Work out the finished part from the listing and answer in its coordinate system (mm). Face numbers are marked on the shaded views. A direction names the side the tool comes from. Give positions to 0.01 mm unless a question says otherwise; leave off trailing zeros. Order: outer loops, then holes, each group sorted by start corner. A loop starts at its lowest first (then second) coordinate and runs counter-clockwise, first axis right, second up.
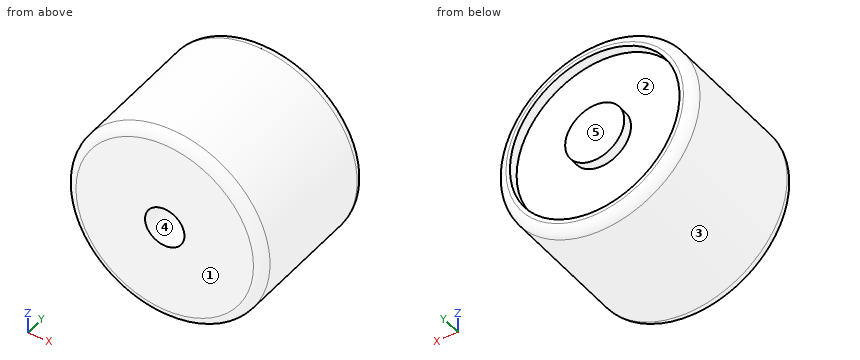
Autodesk Inventor part; units mm, degrees
ref_plane "YZ Plane" through (0, 0, 0) normal (1, 0, 0) x (0, 1, 0)
ref_plane "XZ Plane" through (0, 0, 0) normal (0, 1, 0) x (-1, 0, 0)
ref_plane "XY Plane" through (0, 0, 0) normal (0, 0, 1) x (1, 0, 0)
sketch "Boceto1" plane through (0, 0, 0) normal (0, 1, 0) x (-1, 0, 0)
  circle A0 centre (0, 0) radius 10
  dimension "d0" = 20
extrude "Extrusión1" add sketch "Boceto1" along normal blind 15
sketch "Boceto2" plane through (0, 15, 0) normal (0, 1, 0) x (1, 0, 0)
  circle A0 centre (0, 0) radius 3
  circle A1 centre (0, 0) radius 8.6
  circle A2 centre (0, 0) radius 10
  dimension "d3" = 1.4
  dimension "d4" = 6
extrude "Extrusión2" cut sketch "Boceto2" against normal blind 1 contours A1
sketch "Boceto3" plane through (0, 0, 0) normal (0, -1, 0) x (1, 0, 0)
  circle A0 centre (0, 0) radius 2
  dimension "d7" = 4
extrude "Extrusión3" cut sketch "Boceto3" against normal blind 7.5
fillet "Empalme1" radius 1 2 edges at (10, 0, 0) (10, 15, 0)
properties part number "electromagnet"
1. The part is cut by section D-D (y = 9). Write down the section's boundary in (x, z).
Findings below:
outline: circle Ø20 at (0, 0)
2. Straight lines are drawn through the part: probe 1 along Z at (x, y) = (0, 4.25); probe 2 along Z at (x, y) = (0, 14.7); probe 3 along X at (y, z) = (14.5, -6.25). For each, find the intervals that lie inside material, in ascending order.
Findings below:
probe 1: z = -10 to -2, 2 to 10
probe 2: z = -9.71 to -8.6, -3 to 3, 8.6 to 9.71
probe 3: x = -7.63 to -5.91, 5.91 to 7.63
3. The mould has two halves that part along X. Classify the marked faces 3, 4 and 5: pulls with the +X half, pulls with the -X half, needs draft (parallel to the pull), parting line crosses it, or undercut.
Findings below:
face 3: parting line crosses it
face 4: undercut
face 5: needs draft
4. Given P1, Ø1.5, axis at y = 11, z = 6, coming from the -X side; P2, Ø3, axis at y = 13.5, z = -7.5, coming from the -X side; P3, Ø1.5, axis at y = 11, z = -7, coming from the -X side; P4, Ø10, axis at x = -0.5, z = -6, coming from the +Y side, each flat-ended and moving along its own axis, determine where each tip first touches the part or whether it passes through.
Findings below:
P1: stops at x = -8.51
P2: stops at x = -8
P3: stops at x = -7.81
P4: stops at y = 15
5. The part is cut by section C-C (y = 3.75). Write down the section's boundary in (x, z).
Findings below:
outline: circle Ø20 at (0, 0); hole circle Ø4 at (0, 0)
6. The part is cut by section B-B (x = 0). Write down the section's boundary in (y, z), then the cut area to 3 significant figures.
Findings below:
outline: (0, -9) arc R1 ccw to (1, -10) - (14, -10) arc R1 ccw to (15, -9) - (15, -8.6) - (14, -8.6) - (14, -3) - (15, -3) - (15, 3) - (14, 3) - (14, 8.6) - (15, 8.6) - (15, 9) arc R1 ccw to (14, 10) - (1, 10) arc R1 ccw to (0, 9) - (0, 2) - (7.5, 2) - (7.5, -2) - (0, -2) - close
area: 258 mm2
7. Which of the six approach directions +Z, -Z, +X, -X, +Y, -Y give full straight-line access (tool end or side, diameter ignored) to the marked faces 1 and 2?
Findings below:
face 1: +Z, -Z, +X, -X, -Y
face 2: +Y
8. The part is cut by section A-A (z = 0). Write down the section's boundary in (x, y), then the cut area to 3 significant figures.
Findings below:
outline: (-10, 1) arc R1 ccw to (-9, 0) - (-2, 0) - (-2, 7.5) - (2, 7.5) - (2, 0) - (9, 0) arc R1 ccw to (10, 1) - (10, 14) arc R1 ccw to (9, 15) - (8.6, 15) - (8.6, 14) - (3, 14) - (3, 15) - (-3, 15) - (-3, 14) - (-8.6, 14) - (-8.6, 15) - (-9, 15) arc R1 ccw to (-10, 14) - close
area: 258 mm2
